Design review of the part built by this model. Coordinates are the model's own, in mm. Face numbers are marked on the shaded views. A direction names the side the tool comes from. Give positions to 0.01 mm unless a question says otherwise; leave off trailing zeros. Loops run counter-clockwise (first coordinate to the right, second up) from the corner with the lowest first, then second, coordinate; pieces in that order, holes last. Notation, with made-up numbers: M 4,86.5 L 46,86.5 A13 cw 46,91.5 Z; hole C 10,71 d6. An arc over 180 degrees is marked long. Use CSV: the item, a comma, the result in double quotes.
from build123d import *

# Parameters (mm, degrees)
F0_W      = 20
F0_H      = 40
F0_R      = 3
F1_DEPTH  = 3
F2_W      = 20
F2_H      = 2.5
F3_DEPTH  = 32.5
F4_W      = 20
F4_H      = 2.5
F5_DEPTH  = 80
F6_W      = 20
F6_H      = 30
F6_R      = 6.5
F7_DEPTH  = 2.5
F9_DEPTH  = 2
F11_DEPTH = 2
F12_R     = 6.5


with BuildPart() as f1:
    # F0 (on Front) → F1 (new body)
    with BuildSketch(Plane.XZ):
        Rectangle(F0_W, F0_H)
        with Locations((0, -12.5)):
            Circle(F0_R, mode=Mode.SUBTRACT)
        with Locations((0, -2.5)):
            Circle(F0_R, mode=Mode.SUBTRACT)
    extrude(amount=F1_DEPTH)

    # F2 (on face) → F3 (join)
    with BuildSketch(Plane.XZ.offset(3)):
        with Locations((0, 18.75)):
            Rectangle(F2_W, F2_H)
    extrude(amount=F3_DEPTH)

    # F4 (on face) → F5 (join)
    with BuildSketch(Plane.XY.offset(20)):
        with Locations((0, -34.25)):
            Rectangle(F4_W, F4_H)
    extrude(amount=F5_DEPTH)

    # F6 (on face) → F7 (join)
    with BuildSketch(Plane.XY.offset(100)):
        with Locations((0, -48)):
            Rectangle(F6_W, F6_H)
        with Locations((0, -53)):
            Circle(F6_R, mode=Mode.SUBTRACT)
    extrude(amount=F7_DEPTH)

    # F8 (on Right) → F9 (join)
    with BuildSketch(Plane.YZ):
        Polygon((-34.184523, 89.776114), (-34.184523, 101.863012), (-43.082852, 101.863012), align=None)
    extrude(amount=F9_DEPTH)

    # F10 (on Right) → F11 (join)
    with BuildSketch(Plane.YZ):
        Polygon((-2.943157, 18.818472), (-34.36638, 90.463422), (-34.156892, 18.818472), align=None)
    extrude(amount=F11_DEPTH)

    # F12
    f12_edges = [f1.edges().sort_by_distance(p)[0] for p in [
        (-10, -63, 101.25),
        (10, -63, 101.25),
        (-10, -1.5, -20),
        (10, -1.5, -20),
    ]]
    fillet(f12_edges, radius=F12_R)


solid = f1.part
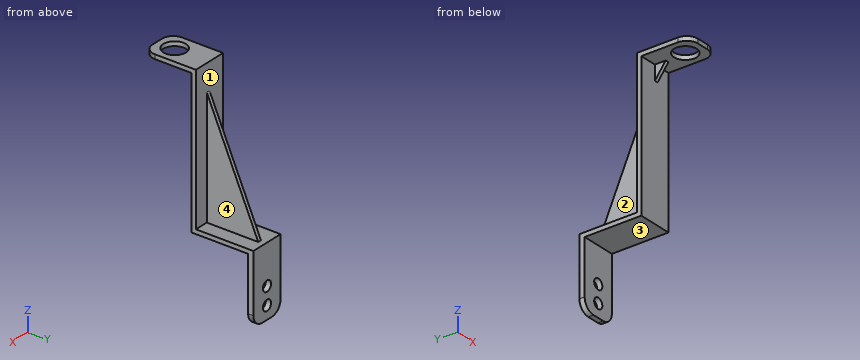
(1) We need section B-B on y = -53. State the section outline as (x, z) points, then the cut area to 3 significant figures.
A:
outline,"M -10,100 L -6.5,100 L -6.5,102.5 L -10,102.5 Z; M 6.5,100 L 10,100 L 10,102.5 L 6.5,102.5 Z"
area,"17.5 mm²"
(2) We need section A-A on z = -2.5. State the section outline as (x, y) points.
A:
outline,"M -10,-3 L -3,-3 L -3,0 L -10,0 Z; M 3,-3 L 10,-3 L 10,0 L 3,0 Z"
(3) Machinability: for the marked faces 1, 2, 3 and 4, which of the approach directions +Z, -Z, +X, -X, +Y, -Y give a long, thin tool a straight path to every point of the face, cutting with its end or side? Answer none if there is none.
A:
face 1,"+Z, +Y"
face 2,"+Z, -X, +Y"
face 3,"-Z, +X, -X, -Y"
face 4,"+Z, +X, +Y"
(4) We need section D-D on z = 79. State the section outline as (x, y) points.
A:
outline,"M -10,-35.5 L 10,-35.5 L 10,-33 L 2,-33 L 2,-29.34 L 0,-29.34 L 0,-33 L -10,-33 Z"
(5) We need section C-C on x = -1.75. State the section outline as (y, z) points, then the cut area to 3 significant figures.
A:
outline,"M -63,100 L -59.26,100 L -59.26,102.5 L -63,102.5 Z; M -46.74,100 L -35.5,100 L -35.5,17.5 L -3,17.5 L -3,-0.06 L 0,-0.06 L 0,20 L -33,20 L -33,102.5 L -46.74,102.5 Z; M -3,-20 L 0,-20 L 0,-14.94 L -3,-14.94 Z; M -3,-10.06 L 0,-10.06 L 0,-4.94 L -3,-4.94 Z"
area,"416 mm²"
(6) Clearance check with flat-ended pins moving along their axes: P1, Ø4, axis at x = -4, y = -37, coming from the -Z side; P2, Ø5, axis at y = -39.5, z = 96.5, coming from the -X side; P3, Ø10, axis at x = -5, z = 56.5, coming from the -Y side. State where each tip first meets the part, or that it passes through.
A:
P1,"z = 17.5"
P2,"x = 0"
P3,"y = -35.5"
(7) Wall thickness on line 1 along Z through (x, y) = (0, -1.2); line 2 along Y through (x, z) = (0, 101.9); line 3 along Z through (x, y) = (-8, -20.5): over which ranges is each line inside the solid? List them lowest first. Write a range as [from, to].
A:
line 1,"[-20, -15.5], [-9.5, -5.5], [0.5, 20]"
line 2,"[-63, -59.5], [-46.5, -33]"
line 3,"[17.5, 20]"
